Geometry check sheet. Reference: the model listing, model coordinates, mm. A direction names the side the tool comes from. Round coordinates to 2 decimals unless told otherwise and drop trailing zeros. Order: outer loops, then holes, each group sorted by start corner. A loop starts at its lowest first (then second) coordinate and runs counter-clockwise, first axis right, second up. Notation, with made-up numbers: M 38,19.5 L 74,19.5 A20 cw 74,54.5 Z; hole C 12.25,41 d6. An arc over 180 degrees is marked long. Answer as a JSON object with one key per item and string values. Group by question number.
Autodesk Inventor part; units mm, degrees
ref_plane "YZ Plane" through (0, 0, 0) normal (1, 0, 0) x (0, 1, 0)
ref_plane "XZ Plane" through (0, 0, 0) normal (0, 1, 0) x (-1, 0, 0)
ref_plane "XY Plane" through (0, 0, 0) normal (0, 0, 1) x (1, 0, 0)
sketch "スケッチ1" plane through (0, 0, 0) normal (0, 1, 0) x (-1, 0, 0)
  arc A0 (182.3045, -62.8657) -> (348.4892, -47.2216) centre (162.2533, 1040.6287) ccw
  arc A1 (135.2834, -62.3282) -> (182.3045, -62.8657) centre (167.871, 731.467) ccw
  arc A2 (49.3906, -47.0603) -> (135.2834, -62.3282) centre (148.588, 261.756) ccw
  arc A3 (0.1309, -22.8654) -> (49.3906, -47.0603) centre (107.173, 132.825) ccw
  arc A4 (-13.3538, -9.7713) -> (0.1309, -22.8654) centre (31.9, 23.342) ccw
  arc A5 (-7.3318, 8.7424) -> (-13.3538, -9.7713) centre (-3.6695, -2.6851) ccw
  arc A6 (12.9042, 11.391) -> (-7.3318, 8.7424) centre (10.0641, -45.5382) ccw
  arc A7 (90.1175, -2.8524) -> (12.9042, 11.391) centre (-1.8944, -285.2401) ccw
  arc A8 (90.1175, -2.8524) -> (94.8834, -4.3943) centre (462.8125, 1140.9603) ccw
  arc A9 (94.8834, -4.3943) -> (348.3291, -45.236) centre (355.7675, 807.7316) ccw
  arc A10 (348.4892, -47.2216) -> (348.3291, -45.236) centre (348.3204, -46.2359) ccw
  circle A11 centre (29.3651, -6.1392) radius 6
  circle A12 centre (239.8151, -50.1371) radius 6
  point P0 (0, 0)
extrude "押し出し1" add sketch "スケッチ1" along normal mid plane 186 contours A1 A2 A3 A4 A5 A6 A7 A8 A9 A10 A0 | A11 | A12
shell "シェル1" thickness 3 outward yes removed faces 2 at (-105.6232, 93, -25.6277) at (-105.6232, -93, -25.6277)
properties part number "GFRP_main"
1) Release check for a two-part mould opening along X. For faces 1 (the cylindrical face through (-264.5, 1.3, -58.3)), 2 (the flat face through (-166, 93, -23)), 3 (the cylindrical face through (-53.08, 1.3, 9.68)) record: +X half, -X half, draft (parallel to the pull), parting line (faces both ways), or undercut.
2) Go/stop test with flat-tipped pins: P1, Ø1, axis at y = -13, z = -40.5, coming from the +X side; P2, Ø1.5, axis at x = -167.5, y = 26, coming from the +Z side; P3, Ø12, axis at x = -32.5, y = 59, coming from the +Z side. Record where each tip stops, or that it passes through.
3) Thickness scan on line 1 along Z through (x, y) = (-111, -2.5); line 2 along Z through (x, y) = (-190.5, -65). Record the ranges inside material, lowest first. Write a range as [from, to].
4) Sectioned sample at A-A (x = -238). Record the boundary of the cut face in (y, z), then the cut area to 3 significant figures.
5) Sectioned sample at B-B (y = 27). Record the boundary of the cut face in (x, z), then the cut area to 3 significant figures.
6) Set-up check for faces 4 (the cylindrical face through (7.259, 1.302, -16.795)), 5 (the cylindrical face through (-218.764, 1.302, -31.155)): record each of +Z, -Z, +X, -X, +Y, -Y from which the full face is reachable in a straight line by a thin tool's end or side.
Final values:
{
 "1": {"face 1": "undercut", "face 2": "draft", "face 3": "-X half"},
 "2": {"P1": "stops at x = -23.68", "P2": "stops at z = -20.99", "P3": "stops at z = 13.41"},
 "3": {"line 1": "z = [-63.44, -60.42], [-9.4, -6.26]", "line 2": "z = [-65.69, -62.69], [-29.11, -26.05]"},
 "4": {"outline": "M -93,-63.45 L 93,-63.45 L 93,-60.45 L -93,-60.45 Z; M -93,-37.1 L 93,-37.1 L 93,-34.07 L -93,-34.07 Z", "area": "1,120 mm^2"},
 "5": {"outline": "M -349,-50.18 A1106.69 ccw -182.36,-65.87 A797.46 ccw -135.16,-65.33 A327.35 ccw -48.47,-49.92 A191.94 ccw 1.57,-25.34 A59.08 ccw 15.77,-11.54 A15 ccw 8.25,11.6 A60 ccw -13.05,14.39 A300 ccw -91.05,0 A1193.01 cw -95.8,-1.54 A850 cw -348.36,-42.24 A4 ccw Z; hole M -348.49,-47.22 A1103.69 ccw -182.3,-62.87 A794.46 ccw -135.28,-62.33 A324.35 ccw -49.39,-47.06 A188.94 ccw -0.13,-22.87 A56.08 ccw 13.35,-9.77 A12 ccw 7.33,8.74 A57 ccw -12.9,11.39 A297 ccw -90.12,-2.85 A1196.01 cw -94.88,-4.39 A853 cw -348.33,-45.24 A1 ccw Z", "area": "2,320 mm^2"},
 "6": {"face 4": "+Y, -Y", "face 5": "+Z, -X, +Y, -Y"}
}
